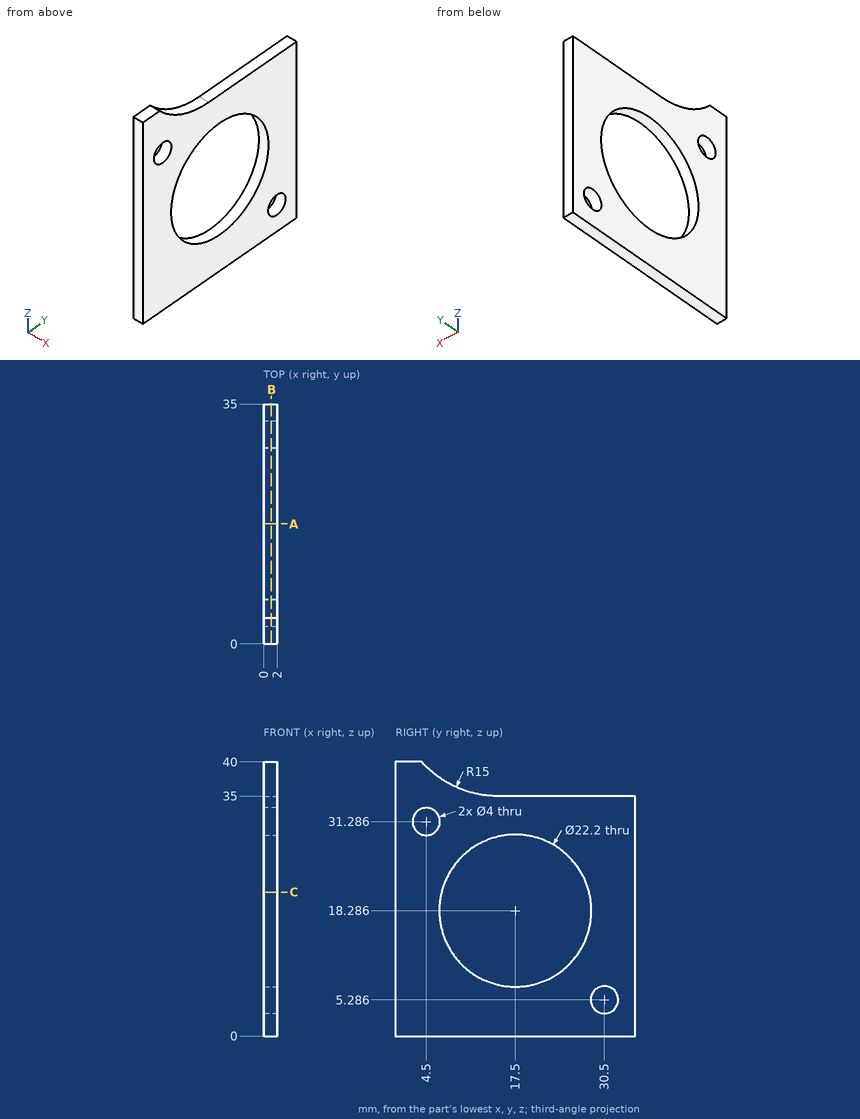
Could you check a few things on this drawing? It's one solid part, dimensions in mm from its lowest x, y, z. Coordinates: 2 decimals unless noted, no trailing zeros. Write each loop counter-clockwise with the first axis right and the second up, starting at its lowest first coordinate (ties: lowest second). Pieces come first, ordered by that corner, then holes. Notation, with made-up numbers: (68.5, -37.5) - (72.5, -37.5) arc R25 cw to (72.5, -7.5) - close; hole circle Ø1 at (-31, 23.25). An arc over 180 degrees is marked (long way). Return JSON: item names as keys, results as strings. Group by question number.
Item 1: I'm going to push flat-ended pins straight in: pin 1 Ø1 at (x, y) = (1.5, 22) entering from +Z; pin 2 Ø5 at (y, z) = (30.5, 5.29) entering from -X; pin 3 Ø18 at (y, z) = (17.5, 18.29) entering from +X. Where does each tip first touch, or does it pass through?
Item 2: If we section it at C-C (z = 21): Write out the boundary of the cut face in (x, y).
Item 3: If we section it at A-A (y = 17.5): Write out the boundary of the cut face in (x, z) (1 decimal).
Item 4: Please list where these lines run through material, in increasing order: probe 1 along Y at (x, z) = (1.85, 31.5); probe 2 along Y at (x, z) = (1.1, 26); probe 3 along Z at (x, y) = (1.8, 9.5) (1 decimal).
Item 5: If we section it at B-B (x = 1.1): Write out the boundary of the cut face in (y, z) (1 decimal).
Return value:
{
 "1": {"pin 1": "stops at z = 35", "pin 2": "stops at x = 0", "pin 3": "passes through"},
 "2": {"outline": "(0, 0) - (2, 0) - (2, 6.74) - (0, 6.74) - close; (0, 28.26) - (2, 28.26) - (2, 35) - (0, 35) - close"},
 "3": {"outline": "(0, 0) - (2, 0) - (2, 7.2) - (0, 7.2) - close; (0, 29.4) - (2, 29.4) - (2, 35) - (0, 35) - close"},
 "4": {"probe 1": "y = 0 to 2.51, 6.49 to 35", "probe 2": "y = 0 to 9.52, 25.48 to 35", "probe 3": "z = 0 to 10.6, 26 to 36"},
 "5": {"outline": "(0, 0) - (35, 0) - (35, 35) - (15, 35) arc R15 cw to (3.8, 40) - (0, 40) - close; hole circle Ø4 at (4.5, 31.3); hole circle Ø22.2 at (17.5, 18.3); hole circle Ø4 at (30.5, 5.3)"}
}
